Build history of the part. All positions in model axes, mm. Give positions to 0.01 mm unless a question says otherwise; leave off trailing zeros. Use a Markdown table: item, result.
from build123d import *

# Parameters (mm, degrees)
F0_W     = 285.75
F0_H     = 31.75
F0_R     = 1.5864569713
F0_R_2   = 1.586899503
F0_R_3   = 1.5819512744
F0_R_4   = 1.5937887431
F0_R_5   = 1.5890160517
F0_R_6   = 1.5902887856
F0_R_7   = 1.5903045613
F0_R_8   = 1.5916317916
F0_R_9   = 3.1764507294
F0_R_10  = 1.5805950388
F0_R_11  = 3.1739361584
F0_R_12  = 1.5864288434
F0_R_13  = 3.1738511752
F0_R_14  = 1.5881643895
F0_R_15  = 1.5816690835
F0_R_16  = 1.5876839815
F0_R_17  = 1.5896769037
F0_R_18  = 3.179191961
F0_R_19  = 1.5871380456
F0_R_20  = 3.1742760912
F0_R_21  = 1.5863757581
F0_R_22  = 3.1737219542
F0_R_23  = 1.5899445862
F0_R_24  = 3.178441897
F0_R_25  = 1.5861913562
F0_R_26  = 1.5855158629
F0_R_27  = 1.5932524318
F0_R_28  = 1.5932021287
F0_R_29  = 1.5925505972
F0_R_30  = 3.1710229814
F0_R_31  = 1.587189734
F0_R_32  = 3.174379468
F0_R_33  = 1.5930868685
F0_R_34  = 3.1741075218
F0_R_35  = 1.5927180648
F0_R_36  = 3.1699091196
F0_R_37  = 1.5849508345
F0_R_38  = 1.5913322568
F0_R_39  = 3.170453012
F0_R_40  = 1.5831664205
F0_R_41  = 3.1707659364
F0_R_42  = 1.589089632
F0_R_43  = 3.1702965498
F0_R_44  = 1.5927776694
F0_R_45  = 3.1687393785
F0_R_46  = 1.5826523304
F0_R_47  = 1.5879751285
F0_R_48  = 1.5841407752
F0_R_49  = 1.583700919
F0_R_50  = 1.5827693871
F0_R_51  = 1.5843354194
F0_R_52  = 1.5863459475
F0_R_53  = 1.589416453
F0_R_54  = 1.5875077881
F0_R_55  = 1.5861476827
F0_R_56  = 1.5892925274
F0_R_57  = 1.5870624762
F0_R_58  = 1.5871828381
F0_R_59  = 1.5926541335
F0_R_60  = 1.589516644
F0_R_61  = 1.5834852409
F1_DEPTH = 1.5875


with BuildPart() as f1:
    # F0 (on Front) → F1 (new body)
    with BuildSketch(Plane.XZ):
        with Locations((70.5032497835, -1.0685799643)):
            Rectangle(F0_W, F0_H)
        with Locations((-56.5036865693, -9.0187799643)):
            Circle(F0_R, mode=Mode.SUBTRACT)
        with Locations((-24.7371103615, -9.0187799643)):
            Circle(F0_R_2, mode=Mode.SUBTRACT)
        with Locations((7.0225620875, -9.0187799643)):
            Circle(F0_R_3, mode=Mode.SUBTRACT)
        with Locations((38.780996576, -9.0187799643)):
            Circle(F0_R_4, mode=Mode.SUBTRACT)
        with Locations((-62.1178604637, -6.6818154435)):
            Circle(F0_R_5, mode=Mode.SUBTRACT)
        with Locations((-50.889512675, -6.6818154435)):
            Circle(F0_R_6, mode=Mode.SUBTRACT)
        with Locations((-64.4426639002, -1.0685799643)):
            Circle(F0_R_7, mode=Mode.SUBTRACT)
        with BuildLine():
            ThreePointArc((-59.6786865693, -1.0685799643), (-56.5036865693, 2.1064200357), (-53.3286865693, -1.0685799643))
            ThreePointArc((-53.3286865693, -1.0685799643), (-56.5036865693, -4.2435799643), (-59.6786865693, -1.0685799643))
        make_face(mode=Mode.SUBTRACT)
        with Locations((-48.5633820081, -1.0685799643)):
            Circle(F0_R_8, mode=Mode.SUBTRACT)
        with Locations((-40.6141579151, -1.0685799643)):
            Circle(F0_R_9, mode=Mode.SUBTRACT)
        with Locations((-32.6759899035, -1.0685799643)):
            Circle(F0_R_10, mode=Mode.SUBTRACT)
        with Locations((-24.7371103615, -1.0685799643)):
            Circle(F0_R_11, mode=Mode.SUBTRACT)
        with Locations((-16.8038876727, -1.0685799643)):
            Circle(F0_R_12, mode=Mode.SUBTRACT)
        with Locations((-8.8644300122, -1.0685799643)):
            Circle(F0_R_13, mode=Mode.SUBTRACT)
        with Locations((1.4070435128, -6.6804702161)):
            Circle(F0_R_14, mode=Mode.SUBTRACT)
        with Locations((12.6380806622, -6.6804702161)):
            Circle(F0_R_15, mode=Mode.SUBTRACT)
        with Locations((64.9241552354, -6.676815734)):
            Circle(F0_R_16, mode=Mode.SUBTRACT)
        with Locations((-0.9215481259, -1.0685799643)):
            Circle(F0_R_17, mode=Mode.SUBTRACT)
        with Locations((7.0225620875, -1.0685799643)):
            Circle(F0_R_18, mode=Mode.SUBTRACT)
        with Locations((14.9631672539, -1.0685799643)):
            Circle(F0_R_19, mode=Mode.SUBTRACT)
        with Locations((22.8988584131, -1.0685799643)):
            Circle(F0_R_20, mode=Mode.SUBTRACT)
        with Locations((30.8337863535, -1.0685799643)):
            Circle(F0_R_21, mode=Mode.SUBTRACT)
        with Locations((38.780996576, -1.0685799643)):
            Circle(F0_R_22, mode=Mode.SUBTRACT)
        with Locations((46.707848087, -1.0685799643)):
            Circle(F0_R_23, mode=Mode.SUBTRACT)
        with Locations((54.6561274678, -1.0685799643)):
            Circle(F0_R_24, mode=Mode.SUBTRACT)
        with Locations((62.6077577472, -1.0685799643)):
            Circle(F0_R_25, mode=Mode.SUBTRACT)
        with Locations((70.5329962075, -9.0187799643)):
            Circle(F0_R_26, mode=Mode.SUBTRACT)
        with Locations((102.2990457714, -9.0187799643)):
            Circle(F0_R_27, mode=Mode.SUBTRACT)
        with Locations((165.7646074891, -9.0187799643)):
            Circle(F0_R_28, mode=Mode.SUBTRACT)
        with Locations((76.1557668447, -6.676815734)):
            Circle(F0_R_29, mode=Mode.SUBTRACT)
        with Locations((70.5329962075, -1.0685799643)):
            Circle(F0_R_30, mode=Mode.SUBTRACT)
        with Locations((78.4771665931, -1.0685799643)):
            Circle(F0_R_31, mode=Mode.SUBTRACT)
        with Locations((86.413115263, -1.0685799643)):
            Circle(F0_R_32, mode=Mode.SUBTRACT)
        with Locations((94.3456701934, -1.0685799643)):
            Circle(F0_R_33, mode=Mode.SUBTRACT)
        with Locations((102.2990457714, -1.0685799643)):
            Circle(F0_R_34, mode=Mode.SUBTRACT)
        with Locations((110.2501451969, -1.0685799643)):
            Circle(F0_R_35, mode=Mode.SUBTRACT)
        with Locations((118.1826815009, -1.0685799643)):
            Circle(F0_R_36, mode=Mode.SUBTRACT)
        with Locations((126.1074505746, -1.0685799643)):
            Circle(F0_R_37, mode=Mode.SUBTRACT)
        with Locations((134.0322196484, -1.0685799643)):
            Circle(F0_R_36, mode=Mode.SUBTRACT)
        with Locations((141.9742777944, -1.0685799643)):
            Circle(F0_R_38, mode=Mode.SUBTRACT)
        with Locations((149.9187275767, -1.0685799643)):
            Circle(F0_R_39, mode=Mode.SUBTRACT)
        with Locations((157.8451916575, -1.0685799643)):
            Circle(F0_R_40, mode=Mode.SUBTRACT)
        with Locations((165.7646074891, -1.0685799643)):
            Circle(F0_R_41, mode=Mode.SUBTRACT)
        with Locations((173.7026423216, -1.0685799643)):
            Circle(F0_R_42, mode=Mode.SUBTRACT)
        with Locations((181.6402077675, -1.0685799643)):
            Circle(F0_R_43, mode=Mode.SUBTRACT)
        with Locations((189.5888373256, -1.0685799643)):
            Circle(F0_R_44, mode=Mode.SUBTRACT)
        with Locations((197.5269839168, -1.0685799643)):
            Circle(F0_R_45, mode=Mode.SUBTRACT)
        with Locations((205.4483443499, -1.0685799643)):
            Circle(F0_R_46, mode=Mode.SUBTRACT)
        with Locations((-62.1173912757, 4.545124742)):
            Circle(F0_R_47, mode=Mode.SUBTRACT)
        with Locations((-50.889512675, 4.5446555149)):
            Circle(F0_R_48, mode=Mode.SUBTRACT)
        with Locations((1.4070435128, 4.5433102875)):
            Circle(F0_R_49, mode=Mode.SUBTRACT)
        with Locations((12.6380806622, 4.5433102875)):
            Circle(F0_R_50, mode=Mode.SUBTRACT)
        with Locations((64.9241552354, 4.549984266)):
            Circle(F0_R_51, mode=Mode.SUBTRACT)
        with Locations((-56.5036865693, 6.8703973666)):
            Circle(F0_R_52, mode=Mode.SUBTRACT)
        with Locations((-24.7371103615, 6.8703973666)):
            Circle(F0_R_53, mode=Mode.SUBTRACT)
        with Locations((7.0225620875, 6.8703973666)):
            Circle(F0_R_54, mode=Mode.SUBTRACT)
        with Locations((38.780996576, 6.8703973666)):
            Circle(F0_R_55, mode=Mode.SUBTRACT)
        with Locations((76.1557668447, 4.549984266)):
            Circle(F0_R_56, mode=Mode.SUBTRACT)
        with Locations((70.5329962075, 6.8703973666)):
            Circle(F0_R_57, mode=Mode.SUBTRACT)
        with Locations((102.2990457714, 6.8703973666)):
            Circle(F0_R_58, mode=Mode.SUBTRACT)
        with Locations((134.0322196484, 6.8703973666)):
            Circle(F0_R_59, mode=Mode.SUBTRACT)
        with Locations((165.7646074891, 6.8703973666)):
            Circle(F0_R_60, mode=Mode.SUBTRACT)
        with Locations((197.5269839168, 6.8703973666)):
            Circle(F0_R_61, mode=Mode.SUBTRACT)
    extrude(amount=F1_DEPTH)


solid = f1.part
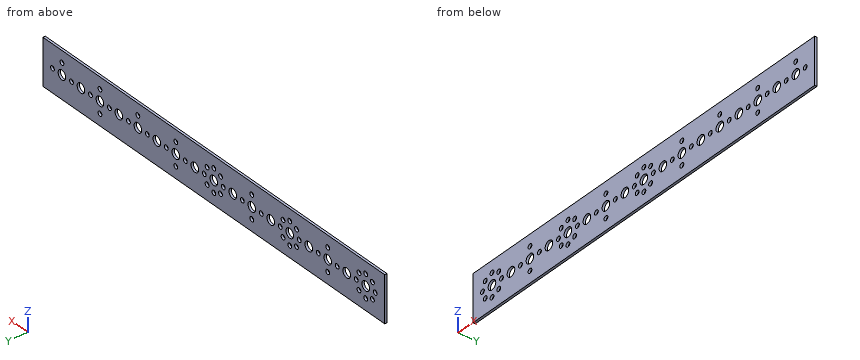
1) Wall check: line 1 (Z direction, x = -56.5, y = -1.35); line 2 (Z direction, x = -57, y = -0.2); line 3 (Z direction, x = 2.5, y = -0.25). Give the ranges that are in metal, low to high. Write a range as from..to.
Computed:
| item | result |
|---|---|
| line 1 | z = -16.94..-10.61, -7.43..-4.24, 2.11..5.28, 8.46..14.81 |
| line 2 | z = -16.94..-10.53, -7.51..-4.2, 2.07..5.36, 8.38..14.81 |
| line 3 | z = -16.94..-7.83, -5.53..3.4, 5.69..14.81 |
2) Slice it at A-A (y = -0.8). State how many separate pieces and enclosed holes the cut face has, and give its area (3 significant figures).
Computed:
| item | result |
|---|---|
| separate pieces | 1 |
| enclosed holes | 63 |
| area | 8,170 mm² |
3) Pin check, flat tip, straight feed: P1, Ø2.5, axis at x = 134.03, z = 6.87, coming from the -Y side. Stop position of the tip, or through.
Computed:
| item | result |
|---|---|
| P1 | passes through |
